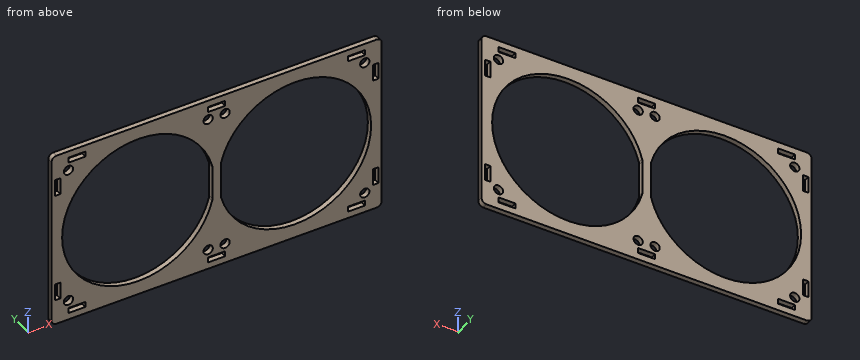
from build123d import *

# Parameters (mm, degrees)
SKETCH1_W           = 195
SKETCH1_H           = 106.45
BOSS_EXTRUDE1_DEPTH = 3.175
SKETCH2_R           = 2.75
CUT_EXTRUDE1_DEPTH  = 112.127095031
FILLET1_R           = 5
FILLET2_R           = 3
SKETCH4_W           = 10
SKETCH4_H           = 3.175
SKETCH4_W_2         = 3.175
SKETCH4_H_2         = 10
CUT_EXTRUDE2_DEPTH  = 112.127095031


with BuildPart() as part:
    # Sketch1 → Boss-Extrude1 (new body)
    with BuildSketch(Plane(origin=(0, 0, 0), x_dir=(1, 0, 0), z_dir=(0, 1, 0))):
        Rectangle(SKETCH1_W, SKETCH1_H)
    extrude(amount=BOSS_EXTRUDE1_DEPTH)

    # Sketch2 → Cut-Extrude1 (cut, through all)
    with BuildSketch(Plane(origin=(0, 3.175, 0), x_dir=(1, 0, 0), z_dir=(0, 1, 0))):
        with Locations(Location((-87.5, 41.25, 0), (0, 0, 270))):
            Circle(SKETCH2_R)
        with Locations(Location((-5, 41.25, 0), (0, 0, 270))):
            Circle(SKETCH2_R)
        with Locations(Location((-5, -41.25, 0), (0, 0, 270))):
            Circle(SKETCH2_R)
        with Locations(Location((-87.5, -41.25, 0), (0, 0, 270))):
            Circle(SKETCH2_R)
        with Locations(Location((5, 41.25, 0), (0, 0, 90))):
            Circle(SKETCH2_R)
        with Locations(Location((5, -41.25, 0), (0, 0, 90))):
            Circle(SKETCH2_R)
        with Locations(Location((87.5, -41.25, 0), (0, 0, 90))):
            Circle(SKETCH2_R)
        with Locations(Location((87.5, 41.25, 0), (0, 0, 90))):
            Circle(SKETCH2_R)
        with BuildLine():
            Line((-2.5, 10.532687216), (-2.5, -10.532687216))
            ThreePointArc((-2.5, -10.532687216), (-91.25, 0), (-2.5, 10.532687216))
        make_face()
        with BuildLine():
            Line((2.5, 10.532687216), (2.5, -10.532687216))
            ThreePointArc((2.5, -10.532687216), (91.25, 0), (2.5, 10.532687216))
        make_face()
    extrude(amount=-CUT_EXTRUDE1_DEPTH, mode=Mode.SUBTRACT)

    # Fillet1
    fillet1_edges = [part.edges().sort_by_distance(p)[0] for p in [
        (-2.5, 1.5875, 10.532687216),
        (-2.5, 1.5875, -10.532687216),
        (2.5, 1.5875, -10.532687216),
        (2.5, 1.5875, 10.532687216),
    ]]
    fillet(fillet1_edges, radius=FILLET1_R)

    # Fillet2
    fillet2_edges = [part.edges().sort_by_distance(p)[0] for p in [
        (-97.5, 1.5875, -53.225),
        (97.5, 1.5875, -53.225),
        (97.5, 1.5875, 53.225),
        (-97.5, 1.5875, 53.225),
    ]]
    fillet(fillet2_edges, radius=FILLET2_R)

    # Sketch4 → Cut-Extrude2 (cut, through all)
    with BuildSketch(Plane.XZ):
        with Locations((-82.5, 47.6375)):
            Rectangle(SKETCH4_W, SKETCH4_H)
        with Locations((0, 47.6375)):
            Rectangle(SKETCH4_W, SKETCH4_H)
        with Locations((82.5, 47.6375)):
            Rectangle(SKETCH4_W, SKETCH4_H)
        with Locations((82.5, -47.6375)):
            Rectangle(SKETCH4_W, SKETCH4_H)
        with Locations((0, -47.6375)):
            Rectangle(SKETCH4_W, SKETCH4_H)
        with Locations((-82.5, -47.6375)):
            Rectangle(SKETCH4_W, SKETCH4_H)
        with Locations((93.8875, -33.05)):
            Rectangle(SKETCH4_W_2, SKETCH4_H_2)
        with Locations((93.8875, 33.05)):
            Rectangle(SKETCH4_W_2, SKETCH4_H_2)
        with Locations((-93.8875, 33.05)):
            Rectangle(SKETCH4_W_2, SKETCH4_H_2)
        with Locations((-93.8875, -33.05)):
            Rectangle(SKETCH4_W_2, SKETCH4_H_2)
    extrude(amount=-CUT_EXTRUDE2_DEPTH, mode=Mode.SUBTRACT)


solid = part.part
Part model, mm, in its own coordinate system. Give positions to 0.01 mm unless a question says otherwise; leave off trailing zeros. Order: outer loops, then holes, each group sorted by start corner. A loop starts at its lowest first (then second) coordinate and runs counter-clockwise, first axis right, second up. Notation, with made-up numbers: (-26, -30.75) -> (-19, -30.75) arc R30 cw to (-19, 6.25) -> close; hole circle Ø9 at (83, 40.25). An arc over 180 degrees is marked (long way). Use one line per item in the form item = value.
(1) Saw through at D-D (x = 56). Write the cut outline in (y, z) (3 decimals).
Solution:
outline = (0, -53.225) -> (3.175, -53.225) -> (3.175, -43.931) -> (0, -43.931) -> close; (0, 43.931) -> (3.175, 43.931) -> (3.175, 53.225) -> (0, 53.225) -> close
(2) Saw through at C-C (z = 0). Write the cut outline in (x, y) (3 decimals).
Solution:
outline = (-97.5, 0) -> (-91.25, 0) -> (-91.25, 3.175) -> (-97.5, 3.175) -> close; (-2.5, 0) -> (2.5, 0) -> (2.5, 3.175) -> (-2.5, 3.175) -> close; (91.25, 0) -> (97.5, 0) -> (97.5, 3.175) -> (91.25, 3.175) -> close
(3) Saw through at A-A (z = -36). Write the cut outline in (x, y) (3 decimals), then the cut area to 3 significant figures.
Solution:
outline = (-97.5, 0) -> (-95.475, 0) -> (-95.475, 3.175) -> (-97.5, 3.175) -> close; (-92.3, 0) -> (-73.25, 0) -> (-73.25, 3.175) -> (-92.3, 3.175) -> close; (-19.25, 0) -> (19.25, 0) -> (19.25, 3.175) -> (-19.25, 3.175) -> close; (73.25, 0) -> (92.3, 0) -> (92.3, 3.175) -> (73.25, 3.175) -> close; (95.475, 0) -> (97.5, 0) -> (97.5, 3.175) -> (95.475, 3.175) -> close
area = 256 mm²
(4) Saw through at B-B (x = -46.25). Write the cut outline in (y, z) (3 decimals), then the cut area to 3 significant figures.
Solution:
outline = (0, -53.225) -> (3.175, -53.225) -> (3.175, -45) -> (0, -45) -> close; (0, 45) -> (3.175, 45) -> (3.175, 53.225) -> (0, 53.225) -> close
area = 52.2 mm²
(5) Drill centre lines: line 1 (X direction, y = 2, z = -1.5) (3 decimals); line 2 (X direction, y = 2.2, z = 47.5); line 3 (Z direction, x = 78.5, y = 2.95) (3 decimals). Where is each one in solid material? Low to high. Write a range as from..to.
Solution:
line_1 = -97.5..-91.225, -2.5..2.5, 91.225..97.5
line_2 = -97.5..-87.5, -77.5..-5, 5..77.5, 87.5..97.5
line_3 = -53.225..-49.225, -46.05..-31.384, 31.384..46.05, 49.225..53.225
